Autodesk Inventor part; units mm, degrees
ref_plane "YZ Plane" through (0, 0, 0) normal (1, 0, 0) x (0, 1, 0)
ref_plane "XZ Plane" through (0, 0, 0) normal (0, 1, 0) x (-1, 0, 0)
ref_plane "XY Plane" through (0, 0, 0) normal (0, 0, 1) x (1, 0, 0)
sketch "Sketch1" plane through (0, 0, 0) normal (0, 0, 1) x (1, 0, 0)
  line L0 (-3.175, -3.175) -> (3.175, -3.175)
  line L1 (3.175, -3.175) -> (3.175, 3.175)
  line L2 (3.175, 3.175) -> (-3.175, 3.175)
  line L3 (-3.175, 3.175) -> (-3.175, -3.175)
  line L4 (-3.175, -3.175) -> (3.175, 3.175) construction
  line L5 (3.175, -3.175) -> (-3.175, 3.175) construction
  circle A0 centre (0, 0) radius 3.81
  point P0 (2.1061, -3.175)
  point P1 (3.175, -2.1061)
  point P2 (3.175, 2.1061)
  point P3 (2.1061, 3.175)
  point P4 (-2.1061, 3.175)
  point P5 (-3.175, 2.1061)
  point P6 (-3.175, -2.1061)
  point P7 (-2.1061, -3.175)
  dimension "d0" = 7.62
  dimension "d1" = 6.35
extrude "Extrusion1" add sketch "Sketch1" against normal blind 12.7 contours A0 L3 L2 L1 L0
sketch "Sketch2" plane through (0, 0, 0) normal (0, 0, 1) x (1, 0, 0)
  arc A0 (-3.175, -2.1061) -> (-2.1061, -3.175) centre (0, 0) ccw construction
  line L0 (-1.5875, -1.5875) -> (1.5875, -1.5875)
  line L1 (1.5875, -1.5875) -> (1.5875, 1.5875)
  line L2 (1.5875, 1.5875) -> (-1.5875, 1.5875)
  line L3 (-1.5875, 1.5875) -> (-1.5875, -1.5875)
  line L4 (-1.5875, -1.5875) -> (1.5875, 1.5875) construction
  line L5 (1.5875, -1.5875) -> (-1.5875, 1.5875) construction
  dimension "d7" = 3.175
extrude "Extrusion2" cut sketch "Sketch2" against normal blind 12.7
fillet "Fillet1" radius 0.254 12 edges at (-1.5875, -1.5875, -6.35) (-1.5875, 1.5875, -6.35) (1.5875, 1.5875, -6.35) (1.5875, -1.5875, -6.35) (2.1061, 3.175, -6.35) (3.175, 2.1061, -6.35) (3.175, -2.1061, -6.35) (2.1061, -3.175, -6.35) (-2.1061, -3.175, -6.35) (-3.175, -2.1061, -6.35) (-3.175, 2.1061, -6.35) (-2.1061, 3.175, -6.35)
properties part number "HS Shaft Adapter Square"
Could you check a few things on this model? Use its own coordinates, in mm. A direction names the side the tool comes from. Give positions to 0.01 mm unless a question says otherwise; leave off trailing zeros. Loops run counter-clockwise (first coordinate to the right, second up) from the corner with the lowest first, then second, coordinate; pieces in that order, holes last. Notation, with made-up numbers: (10.5, 81.5) -> (69.5, 81.5) arc R7 cw to (69.5, 89.5) -> close; hole circle Ø4 at (-12, -28.75). An arc over 180 degrees is marked (long way). Return JSON: item names as keys, results as strings.
Item 1: If we section it at A-A on x = -1: List the corners of the cut face in (y, z) for me (1 decimal).
Geometry results:
{"outline": "(-3.2, -12.7) -> (-1.6, -12.7) -> (-1.6, 0) -> (-3.2, 0) -> close; (1.6, -12.7) -> (3.2, -12.7) -> (3.2, 0) -> (1.6, 0) -> close"}
Item 2: We'd pull the mould along X, two halves only. Please class faces 3 (the flat face through (0, -3.175, -6)), 4 (the cylindrical face through (2.69, -2.7, -6.26)), 5 (the flat face through (-1.588, 0, -6)): +X half, -X half, draft (parallel to the pull), parting line (faces both ways), or undercut.
Geometry results:
{"face 3": "draft", "face 4": "+X half", "face 5": "undercut"}
Item 3: If we section it at D-D on y = 2.5: List the corners of the cut face in (x, z) for me.
Geometry results:
{"outline": "(-2.88, -12.7) -> (2.88, -12.7) -> (2.88, 0) -> (-2.88, 0) -> close"}
Item 4: Which directions (+Z, -Z, +X, -X, +Y, -Y) give clear straight access to the entire face, cutting with the end or side of a thin tool? Please do faces 1 (the cylindrical face through (-2.7, -2.69, -6.26)), 2 (the flat face through (0, 1.588, -6)).
Geometry results:
{"face 1": "+Z, -Z, -X, -Y", "face 2": "+Z, -Z"}
Item 5: I need wall thicknesses on L1, parallel to Y at x = -1, z = -6 (1 decimal); L2, parallel to X at y = -1.5, z = -8.75 (3 decimals). Which ranges of each line are inside material? Lowest first, please. Write a range as from..to.
Geometry results:
{"L1": "y = -3.2..-1.6, 1.6..3.2", "L2": "x = -3.175..-1.525, 1.525..3.175"}
